Geometry: see drawing. Coordinates: mm, zero at the bounding-box minimum. Coordinates: 2 decimals unless noted, no trailing zeros. Write each loop counter-clockwise with the first axis right and the second up, starting at its lowest first coordinate (ties: lowest second). Pieces come first, ordered by that corner, then holes.
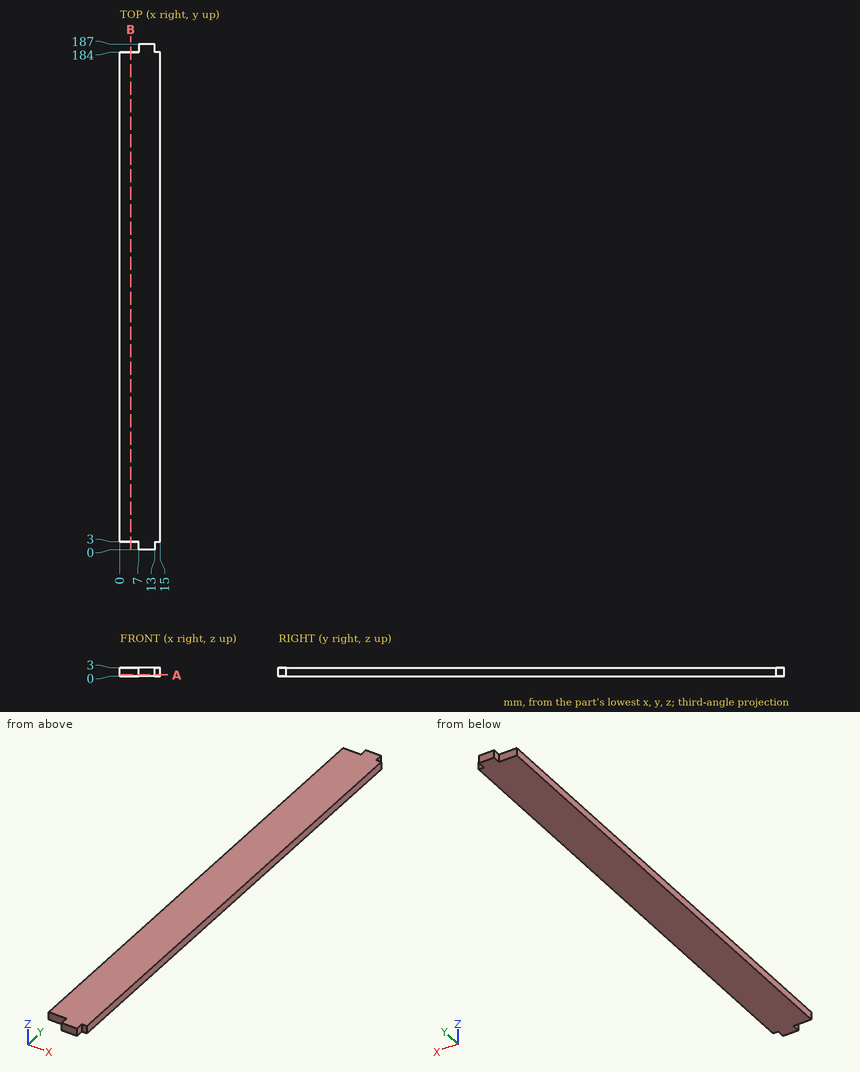
Item 1: Section B-B, the plane x = 4. Output: boundary loops of the cut face in (y, z).
Derived:
outline: (3, 0) - (184, 0) - (184, 3) - (3, 3) - close
Item 2: Material intervals for probe 1 along Y at (x, z) = (6, 0.3), sorted ascending.
Derived:
probe 1: y = 3 to 184
Item 3: Pin query (flat end, axial travel): pin 1 (1.5 mm diameter, centred on y = 1, z = 1.5, fed in from +X); pin 2 (1 mm diameter, centred on x = 2.5, z = 2.5, fed in from +Y); pin 3 (2 mm diameter, centred on x = 6, y = 110.5, fed in from -Z); pin 4 (0.9 mm diameter, centred on x = 4, z = 1, fed in from -Y). Return the tip coordinate at first contact, or that it passes through.
Derived:
pin 1: stops at x = 13
pin 2: stops at y = 184
pin 3: stops at z = 0
pin 4: stops at y = 3
Item 4: Section A-A, the plane z = 0.45. Output: boundary loops of the cut face in (x, y).
Derived:
outline: (0, 3) - (7, 3) - (7, 0) - (13, 0) - (13, 3) - (15, 3) - (15, 184) - (13, 184) - (13, 187) - (7, 187) - (7, 184) - (0, 184) - close
